Part model, mm, in its own coordinate system. A direction names the side the tool comes from. Coordinates: 2 decimals unless noted, no trailing zeros. Order: outer loops, then holes, each group sorted by start corner. A loop starts at its lowest first (then second) coordinate and runs counter-clockwise, first axis right, second up. Notation, with made-up numbers: M 3.5,-24 L 46.5,-24 A22 cw 46.5,-17 Z; hole C 59,41.25 d4. An arc over 180 degrees is marked long. Answer in a Markdown table with one row per item. Add a question column.
from build123d import *

# Parameters (mm, degrees)
CYLINDER048_W                = 5
CYLINDER048_H                = 3
CYLINDER048_ANGLE            = 180
BOX044_W                     = 4
BOX044_H                     = 5
BOX044_DEPTH                 = 2
FUSION002025_PLACEMENT_ANGLE = 180


with BuildPart() as cilindro048:
    # Cylinder048 → Cylinder048 (revolve)
    with BuildSketch(Plane(origin=(-39, 48, 44), x_dir=(-1, 0, 0), z_dir=(0, 1, 0))):
        with Locations((2.5, 1.5)):
            Rectangle(CYLINDER048_W, CYLINDER048_H)
    revolve(axis=Axis((-39, 48, 44), (0, 0, 1)), revolution_arc=CYLINDER048_ANGLE)


with BuildPart() as fusion002025:
    # Box044 → Box044 (new body)
    with BuildSketch(Plane(origin=(-41, 46, 45), x_dir=(1, 0, 0), z_dir=(0, 0, 1))):
        with Locations((2, 2.5)):
            Rectangle(BOX044_W, BOX044_H)
    extrude(amount=BOX044_DEPTH)

    # Fusion002025: union Cilindro048
    add(cilindro048.part)


with BuildPart() as fusion002025_1:
    # Fusion002025 placement: moved
    add(fusion002025.part.moved(Location((-78, 119, 0))).rotate(Axis((-78, 119, 0), (0, 0, 1)), FUSION002025_PLACEMENT_ANGLE))


solid = fusion002025_1.part
(1) 3-axis set-ups, long thin cutter, end or side, ignore diameter. For faces 1 (the cylindrical face through (-39, 76, 46)), 2 (the flat face through (-37, 70, 46)), 3 (the flat face through (-41, 70, 46)), 4 (the flat face through (-39, 68, 46)), 5 (the flat face through (-39, 69, 45)): which of +Z, -Z, +X, -X, +Y, -Y reach the whole face in a straight line?
(2) Slice it at D-D (z = 44.3). List the corners of the cut face in (x, y).
(3) Slice it at C-C (x = -39). List the corners of the cut face in (y, z), and give its area (3 significant figures).
(4) Wall check: line 1 (X direction, y = 69, z = 45.9); line 2 (Z direction, x = -39.75, y = 70.75); line 3 (Y direction, x = -41.5, z = 45.55). Give the ranges that are in metal, low to high.
(5) Drop flat-ended pins along their axis: P1, Ø0.6, axis at y = 70, z = 46.5, coming from the -X side; P2, Ø0.6, axis at y = 70, z = 46, coming from the +X side; P3, Ø1.5, axis at x = -37, y = 70, coming from the -Z side; P4, Ø1, axis at x = -36, y = 69.5, coming from the -Z side. Give the stop position or say it passes through.
(6) Slice it at B-B (y = 69.5). List the corners of the cut face in (x, z), and give its area (3 significant figures).
(7) Slice it at A-A (z = 46.55). List the corners of the cut face in (x, y).
Computed:
| question | item | result |
|---|---|---|
| 1 | face 1 | +Z, -Z, +Y |
| 1 | face 2 | +Z, -Z, +X, -Y |
| 1 | face 3 | +Z, -Z, -X, -Y |
| 1 | face 4 | +Z, -Z, +X, -X, -Y |
| 1 | face 5 | -Z, +X, -X, -Y |
| 2 | outline | M -44,71 L -34,71 A5 ccw Z |
| 3 | outline | M 68,45 L 71,45 L 71,44 L 76,44 L 76,47 L 68,47 Z |
| 3 | area | 21.0 mm^2 |
| 4 | line 1 | x = -41 to -37 |
| 4 | line 2 | z = 45 to 47 |
| 4 | line 3 | y = 71 to 75.33 |
| 5 | P1 | stops at x = -41 |
| 5 | P2 | stops at x = -37 |
| 5 | P3 | stops at z = 45 |
| 5 | P4 | passes through |
| 6 | outline | M -41,45 L -37,45 L -37,47 L -41,47 Z |
| 6 | area | 8.00 mm^2 |
| 7 | outline | M -44,71 L -41,71 L -41,68 L -37,68 L -37,71 L -34,71 A5 ccw Z |
